For this review, take the finished solid that the model builds, in its own axes (mm). A direction names the side the tool comes from. Round coordinates to 2 decimals unless told otherwise and drop trailing zeros. Write each loop counter-clockwise with the first axis right and the second up, starting at its lowest first coordinate (ties: lowest second). Pieces come first, ordered by that corner, then holes.
from build123d import *

# Parameters (mm, degrees)
MODEL_R             = 5.25
BOSS_EXTRUDE1_DEPTH = 6
BOSS_EXTRUDE2_DEPTH = 6
SKETCH3_R           = 60.25
CUT_EXTRUDE1_DEPTH  = 10


with BuildPart() as part:
    # Model → Boss-Extrude1 (new body)
    with BuildSketch(Plane.XZ):
        with BuildLine():
            Line((694.500002921, -169.799850935), (696.999999799, -170.90000032))
            Line((696.999999799, -170.90000032), (694.500002921, -175.370624794))
            Line((694.500002921, -175.370624794), (694.500002921, -216.399998612))
            Line((694.500002921, -216.399998612), (710.5, -216.399998612))
            Line((710.5, -216.399998612), (710.5, -84.4))
            Line((710.5, -84.4), (695.5, -84.4))
            Line((695.5, -84.4), (695.5, -89.4))
            ThreePointArc((695.5, -89.4), (692.807600963, -103.748366696), (685.918459021, -116.61943358))
            ThreePointArc((685.918459021, -116.61943358), (690.782850281, -124.007719547), (694.236343401, -132.151579634))
            ThreePointArc((694.236343401, -132.151579634), (697.533641796, -150.953546779), (694.500002921, -169.799850935))
        make_face()
        with Locations(Location((702.5, -204.808507537, 0), (0, 0, 270))):
            Circle(MODEL_R, mode=Mode.SUBTRACT)
        with Locations(Location((702.5, -99.4, 0), (0, 0, 270))):
            Circle(MODEL_R, mode=Mode.SUBTRACT)
    extrude(amount=BOSS_EXTRUDE1_DEPTH)

    # Sketch2 → Boss-Extrude2 (add)
    with BuildSketch(Plane(origin=(0, 0, 0), x_dir=(1, 0, 0), z_dir=(0, 1, 0))):
        with BuildLine():
            Line((695.5, 84.4), (675.529768986, 104.370231014))
            ThreePointArc((675.529768986, 104.370231014), (681.656132965, 110.674376833), (686.799952909, 117.802890457))
            Line((686.799952909, 117.802890457), (697.045493523, 96.913214697))
            Line((697.045493523, 96.913214697), (695.5, 84.4))
        make_face()
    extrude(amount=-BOSS_EXTRUDE2_DEPTH)

    # Sketch3 → Cut-Extrude1 (cut)
    with BuildSketch(Plane(origin=(0, 0, 0), x_dir=(1, 0, 0), z_dir=(0, 1, 0))):
        with Locations((635.5, 149.4)):
            Circle(SKETCH3_R)
    extrude(amount=-CUT_EXTRUDE1_DEPTH, mode=Mode.SUBTRACT)


solid = part.part
(1) We need section B-B, the plane z = -99.4. Give the boundary of the cut face in (x, y).
Geometry check:
outline: (680.5, -6) - (697.25, -6) - (697.25, 0) - (680.5, 0) - close; (707.75, -6) - (710.5, -6) - (710.5, 0) - (707.75, 0) - close
(2) We need section A-A, the plane x = 702.5. Give the boundary of the cut face in (y, z), and give its area (3 significant figures).
Geometry check:
outline: (-6, -216.4) - (0, -216.4) - (0, -210.06) - (-6, -210.06) - close; (-6, -199.56) - (0, -199.56) - (0, -104.65) - (-6, -104.65) - close; (-6, -94.15) - (0, -94.15) - (0, -84.4) - (-6, -84.4) - close
area: 666 mm2
(3) For line 1 along Z through (x, y) = (702.5, -4.3); line 2 along Z through (x, y) = (698, -5.45); line 3 along X through (y, z) = (-4.55, -186.5), list the stretches that pass through material, from the lowest coordinate up.
Geometry check:
line 1: z = -216.4 to -210.06, -199.56 to -104.65, -94.15 to -84.4
line 2: z = -216.4 to -207.51, -202.1 to -102.1, -96.7 to -84.4
line 3: x = 694.5 to 710.5
(4) For pin 1 Ø12 at (x, z) = (693, -130.5) entering from -Y, flat-tipped, find the tip position at first contact; note if it passes through.
Geometry check:
pin 1: stops at y = -6
(5) For faces 4 (the face through (710.5, -3, -151)), 5 (the face through (694.5, -3, -196)), 6 (the face through (695.73, -2.96, -170.34)), list the 3-axis set-ups (+Z, -Z, +X, -X, +Y, -Y) from which the entire face can be reached by the end or side of a thin tool; tool diameter is ignored.
Geometry check:
face 4: +Z, -Z, +X, +Y, -Y
face 5: -Z, -X, +Y, -Y
face 6: -X, +Y, -Y
(6) We need section D-D, the plane z = -194. Give the boundary of the cut face in (x, y), and give its area (3 significant figures).
Geometry check:
outline: (694.5, -6) - (710.5, -6) - (710.5, 0) - (694.5, 0) - close
area: 96.0 mm2
(7) Mouldability with a two-part tool opening along X and no side actions: class faces 1 (the face through (697.375, -2.958, -98.262)), 2 (the face through (702, -3, -216.4)), 3 (the face through (697.53, -2.96, -150.69)) as pulls with the +X half, pulls with the -X half, needs draft (parallel to the pull), parting line crosses it, or undercut.
Geometry check:
face 1: undercut
face 2: needs draft
face 3: pulls with the -X half
(8) We need section C-C, the plane y = -4.7. State how many separate pieces and enclosed holes the cut face has, and give its area (3 significant figures).
Geometry check:
separate pieces: 1
enclosed holes: 2
area: 2,260 mm2
